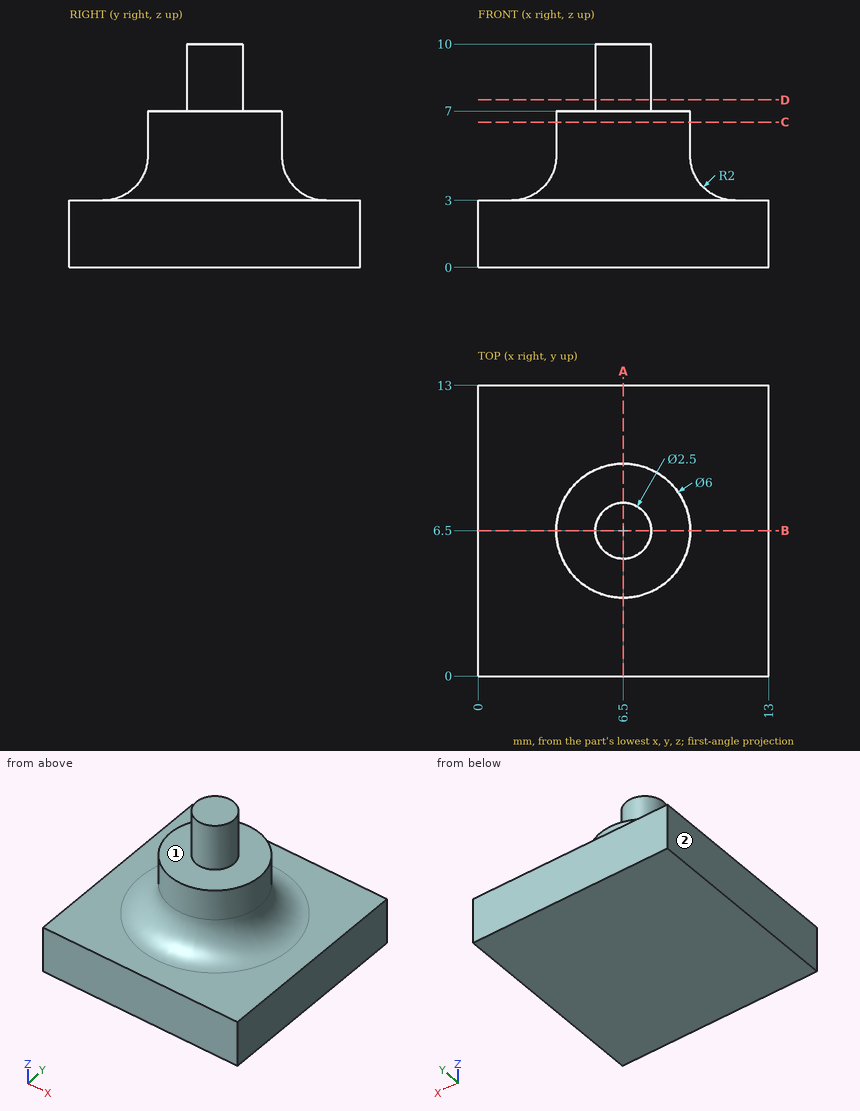
Input: dimensioned drawing with shaded views. Units: mm. Origin: part minimum x, y, z. A direction names the side the tool comes from. Coordinates: 2 decimals unless noted, no trailing zeros. Order: outer loops, then holes, each group sorted by start corner. A loop starts at its lowest first (then second) coordinate and runs counter-clockwise, first axis right, second up.
Item 1: Section query C-C (z = 6.5). Output: boundary loops of the cut face in (x, y), then the cut area to 3 significant figures.
Answer:
outline: circle Ø6 at (6.5, 6.5)
area: 28.3 mm2
Item 2: Contact query for flat-ended pins moving along their axis: P1, Ø5, axis at y = 2.5, z = 8.5, coming from the +X side; P2, Ø4, axis at y = 5, z = 6, coming from the -X side. Output: stop coordinate, or through.
Answer:
P1: stops at x = 8.74
P2: stops at x = 3.4
Item 3: Section query D-D (z = 7.5). Output: boundary loops of the cut face in (x, y), then the cut area to 3 significant figures.
Answer:
outline: circle Ø2.5 at (6.5, 6.5)
area: 4.91 mm2
Item 4: Section query A-A (x = 6.5). Output: boundary loops of the cut face in (y, z).
Answer:
outline: (0, 0) - (13, 0) - (13, 3) - (11.5, 3) arc R2 cw to (9.5, 5) - (9.5, 7) - (7.75, 7) - (7.75, 10) - (5.25, 10) - (5.25, 7) - (3.5, 7) - (3.5, 5) arc R2 cw to (1.5, 3) - (0, 3) - close
Item 5: Access query for the marked faces 1 and 2. Directions: +Z, -Z, +X, -X, +Y, -Y. A direction counts if a zero-diameter tool reaches every point of the face in a straight line with its end or side. Return the directions, or none.
Answer:
face 1: +Z
face 2: +Z, -Z, -X, +Y, -Y
Item 6: Material intervals for line 1 along Z through (x, y) = (11.5, 9); line 2 along Z through (x, y) = (3, 8.5); line 3 along X through (y, z) = (7.25, 6.75), sorted ascending.
Answer:
line 1: z = 0 to 3
line 2: z = 0 to 3.25
line 3: x = 3.6 to 9.4
